Autodesk Inventor part; units mm, degrees
ref_plane "Work Plane1" through (1.525, 0, 0) normal (0, 0, 1) x (1, 0, 0)
ref_plane "YZ Plane" through (0, 0, 0) normal (1, 0, 0) x (0, 1, 0)
ref_plane "XZ Plane" through (0, 0, 0) normal (0, 1, 0) x (-1, 0, 0)
sketch "Sketch1" plane through (0, 0, 0) normal (0, 0, 1) x (1, 0, 0)
  line L0 (0, 16.8) -> (0, 12)
  line L1 (21, 12) -> (75, 12)
  line L2 (75, 12) -> (75, 0)
  line L3 (75, 0) -> (-0.8001, 0)
  line L4 (-15.9601, 0) -> (90.16, 0)
  line L5 (-0.8001, 0) -> (-0.8001, 16.8)
  line L6 (-0.8001, 16.8) -> (0, 16.8)
  line L7 (21, 12) -> (19.1595, 12)
  line L8 (19.1595, 12) -> (0, 12)
  line L9 (0, -3.36) -> (0, 20.16)
  dimension "d0" = 75
  dimension "d1" = 54
  dimension "d2" = 24
  dimension "d9" = 0.8001
  dimension "d10" = 33.6
  dimension "d13" = 1.8404
  dimension "d14" = 24
revolve "Body" add sketch "Sketch1" angle 360 about axis through (75, 0, 0) along (-1, 0, 0)
sketch "Sketch2" plane through (-0.8001, 0, 0) normal (-1, 0, 0) x (0, 0, 1)
  line L0 (0, 20.7846) -> (18, 10.3923)
  line L1 (18, 10.3923) -> (18, -10.3923)
  line L2 (18, -10.3923) -> (0, -20.7846)
  line L3 (0, -20.7846) -> (-18, -10.3923)
  line L4 (-18, -10.3923) -> (-18, 10.3923)
  line L5 (-18, 10.3923) -> (0, 20.7846)
  point P0 (0, 0)
  point P1 (0, 0)
  dimension "d11" = 36
extrude "Head" add sketch "Sketch2" along normal blind 14.2
sketch "Sketch4" plane through (0, 0, 0) normal (0, 0, 1) x (1, 0, 0)
  line L0 (-15.0001, 18) -> (-15.0001, 20.7846)
  line L1 (-15.0001, 20.7846) -> (-13.3924, 20.7846)
  line L2 (-13.3924, 20.7846) -> (-15.0001, 18)
  line L3 (-17.8401, 0) -> (2.0399, 0)
  line L4 (-0.8001, 20.7846) -> (-15.0001, 20.7846)
  line L5 (-15.0001, 10.3923) -> (-15.0001, 20.7846)
  dimension "d5" = 30
  dimension "d19" = 36
revolve "Chamfer1" cut sketch "Sketch4" angle 360 about axis through (-10, 0, 0) along (1, 0, 0)
thread "Thread"
chamfer "Chamfer2" distance 1.8403 distance2 1.8405 1 edges at (75, -12, 0) measured on face at (75, -4.6056, 1.5967)
ref_plane "Work Plane1" through (1.525, 0, 0) normal (0, 0, 1) x (1, 0, 0)
equation "\"d0\" = NLG"
equation "\"d1\" = GEL"
equation "\"d2\" = GD"
equation "\"d10\" = SD2"
equation "\"d14\" = BDM"
equation "\"d11\" = SW"
equation "\"d3\" = KOH - SD"
equation "\"d5\" = ANG1"
equation "\"d19\" = SW0"
equation "\"d15\" = GEL"
equation "\"d6\" = -0.5 * SPD + 0.5 * GD"
equation "\"NLG\" = 75"
equation "\"GD\" = NND"
equation "\"BDM\" = NND"
equation "\"KOH\" = 15"
equation "\"GEL\" = 54"
equation "\"SW\" = 36"
equation "\"SW0\" = SW"
equation "\"SPD\" = NND - 1.2269 * PTC"
equation "\"SD2\" = 33.6"
equation "\"SD\" = 0.8"
equation "\"ANG1\" = 30deg"
equation "\"GAL\" = 0.61345 * PTC"
equation "\"GUL\" = 0.61345 * PTC"
equation "\"RR\" = 0.8"
equation "\"WFT\" = SD"
equation "\"GD1\" = THREADDIA - 1.2269 * PTC"
equation "\"THREADDIA\" = 24"
equation "\"SDH\" = 33.6"
equation "\"TOA\" = 30deg"
equation "\"FAWI\" = 45deg"
equation "\"PTC\" = 3"
equation "\"NND\" = 24"
equation "\"E0\" = 1.155 * SW"
properties part number "Bolt M24x75-8.8-A PN-85/M-82101" material "Steel, Mild"
CAD build for the part. Positions are in the model's coordinates, mm. A direction names the side the tool comes from. Round coordinates to 2 decimals unless told otherwise and drop trailing zeros. Write each loop counter-clockwise with the first axis right and the second up, starting at its lowest first coordinate (ties: lowest second). Pieces come first, ordered by that corner, then holes. Notation, with made-up numbers: (-18.5, -5) - (33.5, -5) arc R15 cw to (33.5, 21) - close; hole circle Ø11 at (-40, 59). An arc over 180 degrees is marked (long way). Write item = value, one per line. Start each with the question number.
Q1. Which spindle directions (+Z, -Z, +X, -X, +Y, -Y) get a long thin tool onto all of the face, cutting with end or side? Do faces 1 (the flat face through (-7.801, -15.661, -8.874)), 2 (the cylindrical face through (36.07, -11.99, -0.53)). Say none if no direction does.
Q2. Probe L1, parallel to X at y = -17, z = 2.5; L2, parallel to X at y = -3, z = -12; L3, parallel to Z at x = 12, y = 7. List the from-to ranges inside material, lowest first. Write a range as from..to.
Q3. Band-saw the part on A-A (x = 12). Give the cut face in (y, z).
Q4. Drop flat-ended pins along their axis: pin 1 (1 mm diameter, centred on x = 19, y = 6.5, fed in from +Z); pin 2 (5 mm diameter, centred on x = -3.5, y = -13, fed in from +Z); pin 3 (5 mm diameter, centred on x = 29.5, y = -9.5, fed in from -Z). Give the stop position or say it passes through.
Answers below:
q1.face_1 = -Z, +X, -X, -Y
q1.face_2 = +X
q2.L1 = -15..-0.8
q2.L2 = -15..0
q2.L3 = -9.75..9.75
q3.outline = circle Ø24 at (0, 0)
q4.pin_1 = 10.39
q4.pin_2 = 17.81
q4.pin_3 = -9.75
